For this review, take the finished solid that the model builds, in its own axes (mm). A direction names the side the tool comes from. Give positions to 0.01 mm unless a question says otherwise; leave off trailing zeros. Write each loop counter-clockwise with the first axis right and the second up, starting at its lowest first coordinate (ties: lowest second). Pieces come first, ordered by that corner, then holes. Notation, with made-up numbers: M -39,14.25 L 8,14.25 A25 ccw 8,43.25 Z; hole C -19.75,89 d5. An arc over 180 degrees is marked long. Use one line per item in the form item = value. Start each with the question number.
Q1. Consider section C-C on x = 6. Write out the cut boundary in (y, z).
Q2. Clearance check with flat-ended pins moving along their axes: pin 1 Ø1.5 at (x, y) = (5.5, -2.5) entering from +Z; pin 2 Ø0.6 at (x, z) = (27.5, -2.5) entering from -Y; pin 3 Ø2 at (y, z) = (-4.5, -2) entering from +X. State where each tip first meets the part, or that it passes through.
Q3. Consider section D-D on z = 1.85. Write out the cut boundary in (x, y), and give its area (3 significant figures).
Q4. Consider section B-B on y = -8. Write out the cut boundary in (x, z), and give its area (3 significant figures).
Q5. Mouldability with a two-part tool opening along Y and no side actions: class faces 6 (the flat face through (20, -7, -2)), 7 (the flat face through (19.4, -13.3, -0.7)), 8 (the cylindrical face through (16.729, 11.223, -0.042)), 9 (the flat face through (0.7, 16.4, -0.7)) as released by +Y, released by -Y, zero draft, split by the parting line, or undercut.
Q6. For probe 1 along Y at (x, z) = (17, -1); probe 2 along Y at (x, z) = (36, 1.7); probe 3 along X at (y, z) = (12, -0.15), list the stretches that pass through material, from the lowest coordinate up. Write a range as [from, to].
Q7. Consider section A-A on x = 36. Write out the cut boundary in (y, z).
Q8. Tool access review of faces 1 (the flat face through (39.5, 16.5, -2)), 2 (the flat face through (0.5, -13.5, -2)), 3 (the cylindrical face through (33.003, 12.575, 1.479)), 4 (the flat face through (29.9, 0.5, -0.5)), 5 (the flat face through (30, 0, -2)): name each direction out of +Z, -Z, +X, -X, +Y, -Y from which nothing blocks a thin tool from reaching the whole face with its end or side.
```python
from build123d import *

# Parameters (mm, degrees)
F0_W     = 20
F0_H     = 14
F0_R     = 2.7148316461
F0_R_2   = 3
F0_R_3   = 1.25
F1_DEPTH = 3
F2_R     = 5
F2_R_2   = 2.7148316461
F3_DEPTH = 1
F4_DEPTH = 3
F5_SIZE  = 0.99999


# Not quite as in the source:
# - a fillet or chamfer is up to 0.001 mm smaller than in the source, because OpenCascade refuses the exact size


with BuildPart() as f1:
    # F0 (on Top) → F1 (new body)
    with BuildSketch(Plane.XY):
        with Locations((10, -7)):
            Rectangle(F0_W, F0_H)
        with Locations((10, -7)):
            Circle(F0_R, mode=Mode.SUBTRACT)
        Polygon((0, 17), (0, 0), (20, 0), (40, 0), (40, 17), align=None)
        with Locations((17, 12.44318299)):
            Circle(F0_R_2, mode=Mode.SUBTRACT)
        with Locations((36, 12.44318299)):
            Circle(F0_R_2, mode=Mode.SUBTRACT)
        with Locations((36, 12.44318299)):
            Circle(F0_R_2)
        with Locations((36, 12.44318299)):
            Circle(F0_R_3, mode=Mode.SUBTRACT)
        with Locations((17, 12.44318299)):
            Circle(F0_R_2)
        with Locations((17, 12.44318299)):
            Circle(F0_R_3, mode=Mode.SUBTRACT)
    extrude(amount=-F1_DEPTH)

    # F2 (on face) → F3 (cut)
    with BuildSketch(Plane.XY):
        with Locations((10, -7)):
            Circle(F2_R)
        with Locations((10, -7)):
            Circle(F2_R_2, mode=Mode.SUBTRACT)
    extrude(amount=-F3_DEPTH, mode=Mode.SUBTRACT)

    # F0 (on Top) → F4 (join)
    with BuildSketch(Plane.XY):
        with Locations((17, 12.44318299)):
            Circle(F0_R_2)
        with Locations((17, 12.44318299)):
            Circle(F0_R_3, mode=Mode.SUBTRACT)
        with Locations((36, 12.44318299)):
            Circle(F0_R_2)
        with Locations((36, 12.44318299)):
            Circle(F0_R_3, mode=Mode.SUBTRACT)
    extrude(amount=F4_DEPTH)

    # F5 (size 1 in the source; OpenCascade refuses exactly that, so slightly less here)
    f5_edges = [f1.edges().sort_by_distance(p)[0] for p in [
        (0, 1.5, 0),
        (10, -14, 0),
        (20, -7, 0),
        (30, 0, 0),
        (40, 8.5, 0),
        (20, 17, 0),
        (40, 0, -1.5),
        (40, 17, -1.5),
        (20, -14, -1.5),
        (0, 17, -1.5),
        (0, -14, -1.5),
        (20, 0, -1.5),
    ]]
    chamfer(f5_edges, length=F5_SIZE)


solid = f1.part
```
Working result:
q1.outline = M -14,-3 L 17,-3 L 17,-1 L 16,0 L -4,0 L -4,-1 L -10,-1 L -10,0 L -13,0 L -14,-1 Z
q2.pin_1 = 0
q2.pin_2 = 0
q2.pin_3 = 20
q3.outline = C 17,12.44 d6; C 36,12.44 d6; hole C 17,12.44 d2.5; hole C 36,12.44 d2.5
q3.area = 46.7 mm²
q4.outline = M 0,-3 L 7.48,-3 L 7.48,-1 L 5.1,-1 L 5.1,0 L 1,0 L 0,-1 Z; M 12.52,-3 L 20,-3 L 20,-1 L 19,0 L 14.9,0 L 14.9,-1 L 12.52,-1 Z
q4.area = 39.1 mm²
q5.face_6 = zero draft
q5.face_7 = released by -Y
q5.face_8 = undercut
q5.face_9 = released by +Y
q6.probe_1 = [-14, 11.19], [13.69, 17]
q6.probe_2 = [9.44, 11.19], [13.69, 15.44]
q6.probe_3 = [0.85, 15.83], [18.17, 34.83], [37.17, 39.15]
q7.outline = M 0,-3 L 11.19,-3 L 11.19,3 L 9.44,3 L 9.44,0 L 1,0 L 0,-1 Z; M 13.69,-3 L 17,-3 L 17,-1 L 16,0 L 15.44,0 L 15.44,3 L 13.69,3 Z
q8.face_1 = +Z, -Z, +X, +Y
q8.face_2 = +Z, -Z, -X, -Y
q8.face_3 = +Z
q8.face_4 = +Z, +X, -Y
q8.face_5 = +Z, -Z, +X, -Y
